Can you work these out from the drawing? Everything is in mm from the part's minimum corner. Coordinates: 2 decimals unless noted, no trailing zeros. Order: outer loops, then holes, each group sorted by start corner. A loop starts at its lowest first (then second) coordinate and runs counter-clockwise, first axis right, second up. Notation, with made-up numbers: (23, -13) -> (65, -13) arc R17 ccw to (65, 12) -> close; hole circle Ø10 at (32.25, 0.5). An arc over 180 degrees is marked (long way). Put each result on its own line as item: value. Start each with the question number.
Q1. Will these pins go through, and if not, where does the flat tip stop? pin 1 (1.5 mm diameter, centred on x = 10, y = 6.5, fed in from -Z); pin 2 (2 mm diameter, centred on y = 2, z = 3, fed in from +X); pin 3 (4 mm diameter, centred on y = 14.5, z = 7.5, fed in from +X).
Q2. Please list where these lines run through material, in increasing order: line 1 along X through (y, z) = (5.5, 6); line 2 along X through (y, z) = (12.75, 6); line 3 along Z through (x, y) = (6.75, 4.5).
Q3. If we section it at D-D (y = 3.5): Please give me the cut outline in (x, z), and give its area (3 significant figures).
Q4. If we section it at C-C (y = 6.5): Please give me the cut outline in (x, z), and give its area (3 significant figures).
Q5. We'd pull the mould along X, two halves only. Please class the marked faces 1, 2 and 3: +X half, -X half, draft (parallel to the pull), parting line (faces both ways), or undercut.
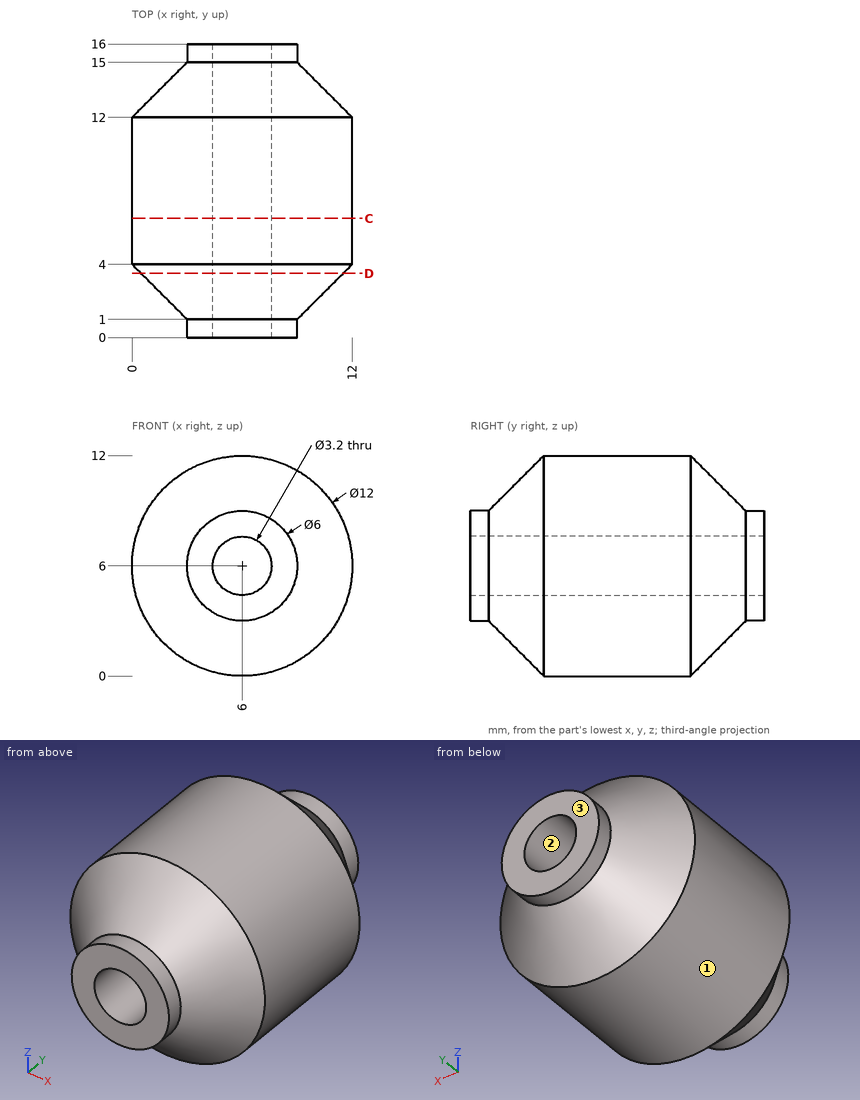
The answers:
1. pin 1: z = 0.96
1. pin 2: x = 10.18
1. pin 3: x = 11.35
2. line 1: 0 to 4.4, 7.6 to 12
2. line 2: 0.75 to 4.4, 7.6 to 11.25
2. line 3: 0.05 to 4.59, 7.41 to 11.95
3. outline: circle Ø11 at (6, 6); hole circle Ø3.2 at (6, 6)
3. area: 87.0 mm^2
4. outline: circle Ø12 at (6, 6); hole circle Ø3.2 at (6, 6)
4. area: 105 mm^2
5. face 1: parting line
5. face 2: undercut
5. face 3: draft
